The figure shows three views and two pictorial views of one solid part (mm, origin at its lowest corner). Answer the questions. Coordinates: 2 decimals unless noted, no trailing zeros. Loops run counter-clockwise (first coordinate to the right, second up) from the corner with the lowest first, then second, coordinate; pieces in that order, holes last. Notation, with made-up numbers: M 7.25,52.5 L 60.25,52.5 A21 ccw 60.25,58.5 Z; hole C 37.5,85.25 d9. An arc over 180 degrees is marked long. Answer in a Markdown table with one row per item. Add a question column.
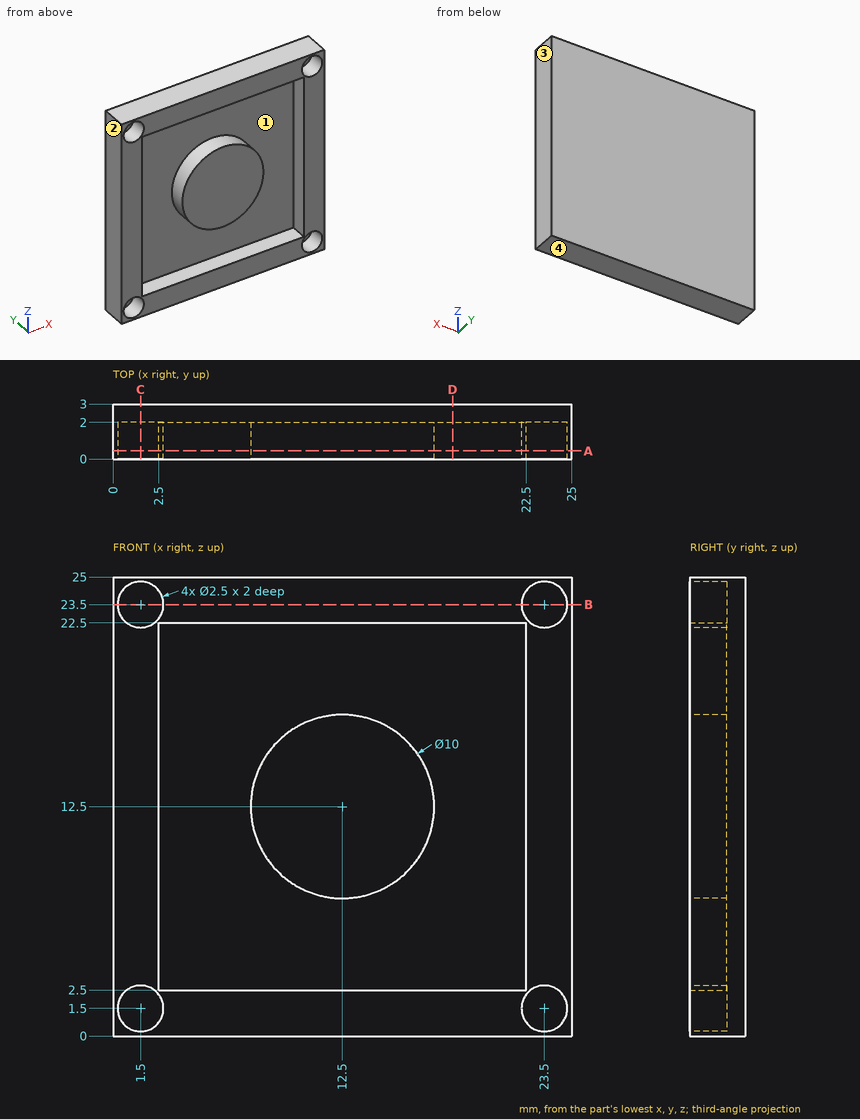
(1) A cutting plane is placed at A-A (y = 0.45). Give the vertices of the cut face in (x, z), plus the area to 3 significant figures.
(2) A cutting plane is placed at C-C (x = 1.5). Give the vertices of the cut face in (y, z), plus the area to 3 significant figures.
(3) The mould has two halves that part along X. Classify the marked faces 1, 2, 3 and 4: released by +X, released by -X, zero draft, split by the parting line, or undercut.
(4) This flat-tipped pin is pushed along its axis until it touches: pin 1 (0.8 mm diameter, centred on x = 2, z = 23.5, fed in from -Y). Where does it stop, or does it pass through?
(5) Straight lines are drawn through the part: line 1 (Z direction, x = 23.5, y = 1.1); line 2 (Z direction, x = 3, y = 1.5). For each, find the intervals that lie inside material, in ascending order.
(6) A cutting plane is placed at B-B (z = 23.5). Give the vertices of the cut face in (x, y).
(7) A cutting plane is placed at D-D (x = 18.5). Give the vertices of the cut face in (y, z), plus the area to 3 significant figures.
Solved:
| question | item | result |
|---|---|---|
| 1 | outline | M 0,0 L 25,0 L 25,25 L 0,25 Z; C 12.5,12.5 d10; hole C 1.5,1.5 d2.5; hole C 1.5,23.5 d2.5; hole M 2.5,2.5 L 22.5,2.5 L 22.5,22.5 L 2.5,22.5 Z; hole C 23.5,1.5 d2.5; hole C 23.5,23.5 d2.5 |
| 1 | area | 284 mm² |
| 2 | outline | M 0,0 L 3,0 L 3,25 L 0,25 L 0,24.75 L 2,24.75 L 2,22.25 L 0,22.25 L 0,2.75 L 2,2.75 L 2,0.25 L 0,0.25 Z |
| 2 | area | 65.0 mm² |
| 3 | face 1 | undercut |
| 3 | face 2 | released by -X |
| 3 | face 3 | released by +X |
| 3 | face 4 | zero draft |
| 4 | pin 1 | stops at y = 2 |
| 5 | line 1 | z = 0 to 0.25, 2.75 to 22.25, 24.75 to 25 |
| 5 | line 2 | z = 0 to 2.5, 22.5 to 25 |
| 6 | outline | M 0,0 L 0.25,0 L 0.25,2 L 2.75,2 L 2.75,0 L 22.25,0 L 22.25,2 L 24.75,2 L 24.75,0 L 25,0 L 25,3 L 0,3 Z |
| 7 | outline | M 0,0 L 3,0 L 3,25 L 0,25 L 0,22.5 L 2,22.5 L 2,2.5 L 0,2.5 Z |
| 7 | area | 35.0 mm² |
